Design review of the part built by this model. Coordinates are the model's own, in mm. Face numbers are marked on the shaded views. A direction names the side the tool comes from. Coordinates: 2 decimals unless noted, no trailing zeros. Order: outer loops, then holes, each group sorted by start corner. A loop starts at its lowest first (then second) coordinate and runs counter-clockwise, first axis right, second up. Notation, with made-up numbers: (72.25, 58.25) - (111.25, 58.25) arc R25 cw to (111.25, 81.25) - close; hole circle Ø9 at (76.5, 39.25). An arc over 180 degrees is marked (long way). Write item = value, one per line. Start each with the question number.
```python
from build123d import *

# Parameters (mm, degrees)
SKETCH_1_W          = 16
SKETCH_1_H          = 26
EXTRUDE_1_DEPTH     = 4
SKETCH_2_W          = 16
SKETCH_2_H          = 4
EXTRUDE_2_DEPTH     = 20
SKETCH_3_W          = 16
SKETCH_3_H          = 12
EXTRUDE_3_DEPTH     = 2
FILLET_2_R          = 4
FILLET_START        = -8
FILLET_3_DEPTH      = 16
SKETCH_4_W          = 10
SKETCH_4_H          = 6
CUT_EXTRUDE_2_DEPTH = 34.520714063
CUT_EXTRUDE_3_DEPTH = 4
CUT_EXTRUDE_4_DEPTH = 2


with BuildPart() as part:
    # Эскиз1 → Бобышка-Вытянуть1 (new body)
    with BuildSketch(Plane.XY):
        Rectangle(SKETCH_1_W, SKETCH_1_H)
    extrude(amount=EXTRUDE_1_DEPTH)

    # Эскиз2 → Бобышка-Вытянуть2 (add)
    with BuildSketch(Plane.XY.offset(4)):
        with Locations((0, -10.991777356)):
            Rectangle(SKETCH_2_W, SKETCH_2_H)
    extrude(amount=EXTRUDE_2_DEPTH)

    # Эскиз3 → Бобышка-Вытянуть3 (add)
    with BuildSketch(Plane(origin=(0, 0, 0), x_dir=(-1, 0, 0), z_dir=(0, 0, -1))):
        with Locations((0, 7)):
            Rectangle(SKETCH_3_W, SKETCH_3_H)
    extrude(amount=EXTRUDE_3_DEPTH)

    # Скругление2
    fillet_2_edges = [part.edges().sort_by_distance(p)[0] for p in [
        (0, -8.991777356, 4),
    ]]
    fillet(fillet_2_edges, radius=FILLET_2_R)

    # Скругление3: read off the stored shape, not the designer's step
    # Скругление3 outline → Скругление3 (cut)
    with BuildSketch(Plane.YZ.offset(FILLET_START)):
        with BuildLine():
            ThreePointArc((-8.991777356, 0), (-11.820204481, 1.171572875), (-12.991777356, 4))
            Line((-12.991777356, 4), (-13, 4))
            Line((-13, 4), (-13, 0))
            Line((-13, 0), (-8.991777356, 0))
        make_face()
    extrude(amount=FILLET_3_DEPTH, mode=Mode.SUBTRACT)

    # Эскиз4 → Вырез-Вытянуть2 (cut, through all)
    with BuildSketch(Plane(origin=(0, -8.991777356, 0), x_dir=(1, 0, 0), z_dir=(0, 1, 0))):
        with Locations((0, -21)):
            Rectangle(SKETCH_4_W, SKETCH_4_H)
    extrude(amount=-CUT_EXTRUDE_2_DEPTH, mode=Mode.SUBTRACT)

    # Эскиз5 → Вырез-Вытянуть3 (cut)
    with BuildSketch(Plane.XY.offset(4)):
        with BuildLine():
            Line((-5, 13), (-5, 8))
            ThreePointArc((-5, 8), (0, 3), (5, 8))
            Line((5, 8), (5, 13))
            Line((5, 13), (-5, 13))
        make_face()
    extrude(amount=-CUT_EXTRUDE_3_DEPTH, mode=Mode.SUBTRACT)

    # Эскиз7 → Вырез-Вытянуть4 (cut)
    with BuildSketch(Plane.XY):
        with BuildLine():
            Line((-2.5, 13), (-2.5, 8))
            ThreePointArc((-2.5, 8), (0, 5.5), (2.5, 8))
            Line((2.5, 8), (2.5, 13))
            Line((2.5, 13), (-2.5, 13))
        make_face()
    extrude(amount=-CUT_EXTRUDE_4_DEPTH, mode=Mode.SUBTRACT)


solid = part.part
```
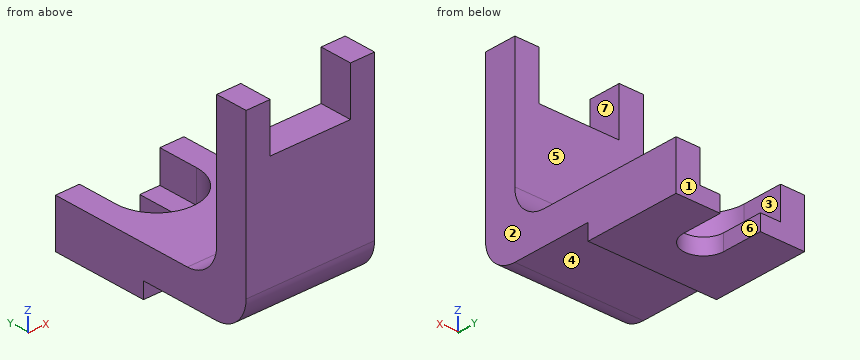
Item 1: Add section D-D on y = 2.5. Give the boundary of the cut face in (x, z).
Item 2: For the marked faces 4, 5, 6 and 7, list the 3-axis set-ups (+Z, -Z, +X, -X, +Y, -Y) from which the entire face can be reached by the end or side of a thin tool; tool diameter is ignored.
Item 3: Mouldability with a two-part tool opening along X and no side actions: class the marked faces 1, 2 and 3 as +X half, -X half, draft (parallel to the pull), parting line (faces both ways), or undercut.
Item 4: Add section B-B on x = 0. Give the boundary of the cut face in (y, z).
Item 5: For line 1 (X direction, y = -10.5, z = 20.25); line 2 (Z direction, x = -6.25, y = 9.25); line 3 (Z direction, x = 0.25, y = -3), list the stretches that pass through material, from the lowest coordinate up.
Item 6: For P1, Ø3, axis at x = 2, y = 7.5, coming from the +Z side; P2, Ø5, axis at x = 3, y = 1, coming from the +Z side; P3, Ø2, axis at x = 1, y = -11, coming from the +Z side, all flat-tipped, find the tip position at first contact; note any pin that passes through.
Item 7: Add section C-C on z = 12.5. Give the boundary of the cut face in (x, y), plus the area to 3 significant figures.
Item 8: Add section A-A on y = 8.75. Give the boundary of the cut face in (x, z).
Worked out:
q1.outline = (-8, -2) - (8, -2) - (8, 4) - (-8, 4) - close
q2.face_4 = -Z, +X, -X, -Y
q2.face_5 = +Z, +X, -X, +Y
q2.face_6 = +Z, -Z, +Y
q2.face_7 = +Z, +Y, -Y
q3.face_1 = draft
q3.face_2 = +X half
q3.face_3 = undercut
q4.outline = (-12.99, 4) arc R4 ccw to (-8.99, 0) - (1, 0) - (1, -2) - (5.5, -2) - (5.5, 0) - (3, 0) - (3, 4) - (-4.99, 4) arc R4 cw to (-8.99, 8) - (-8.99, 18) - (-12.99, 18) - close
q5.line_1 = -8 to -5, 5 to 8
q5.line_2 = -2 to 4
q5.line_3 = 0 to 4
q6.P1 = 0
q6.P2 = 4
q6.P3 = 18
q7.outline = (-8, -12.99) - (8, -12.99) - (8, -8.99) - (-8, -8.99) - close
q7.area = 64.0 mm2
q8.outline = (-8, -2) - (-2.5, -2) - (-2.5, 0) - (-5, 0) - (-5, 4) - (-8, 4) - close; (2.5, -2) - (8, -2) - (8, 4) - (5, 4) - (5, 0) - (2.5, 0) - close
